```python
from build123d import *

# Parameters (mm, degrees)
CUT_EXTRUDE_1_DEPTH = 2
FILLET_1_R          = 0.2


with BuildPart() as part:
    # 草图1 → 旋转1 (revolve)
    with BuildSketch(Plane.XY):
        Polygon((0, 0), (0, 3.5), (3.5, 3.5), (3.5, 2), (7.5, 2), (7.5, 1.5), (13.5, 1.5), (13.5, 0), align=None)
    revolve(axis=Axis((13.5, 0, 0), (-1, 0, 0)))

    # 草图2 → 切除-拉伸1 (cut)
    with BuildSketch(Plane.ZY):
        Polygon((1.5, 0.866025404), (0, 1.732050808), (-1.5, 0.866025404), (-1.5, -0.866025404), (0, -1.732050808), (1.5, -0.866025404), align=None)
    extrude(amount=-CUT_EXTRUDE_1_DEPTH, mode=Mode.SUBTRACT)

    # 圆角1
    fillet_1_edges = [part.edges().sort_by_distance(p)[0] for p in [
        (3.5, -3.5, 0),
        (0, -3.5, 0),
    ]]
    fillet(fillet_1_edges, radius=FILLET_1_R)


solid = part.part
```
Here's how the part is built. I have some questions about the finished solid (model axes, mm). A direction names the side the tool comes from. Round coordinates to 2 decimals unless told otherwise and drop trailing zeros. Loops run counter-clockwise (first coordinate to the right, second up) from the corner with the lowest first, then second, coordinate; pieces in that order, holes last. Notation, with made-up numbers: (54, 64) -> (75, 64) arc R25 ccw to (75, 103) -> close; hole circle Ø6 at (1.5, 66.25). An arc over 180 degrees is marked (long way). Answer as CSV lines item,"result". Start each with the question number.
1. Imagine slicing it at A-A on x = 1. Write out the boundary of the cut face in (y, z), plus the area to 3 significant figures.
2. I'm going to push flat-ended pins straight in: P1, Ø4, axis at x = 12, y = -1, coming from the +Z side; P2, Ø1, axis at y = 1.5, z = 1.5, coming from the +X side; P3, Ø3, axis at x = 10, y = 1, coming from the -Z side. Where does each tip first touch, or does it pass through?
3. I need wall thicknesses on probe 1 along X at (y, z) = (-0.75, -1.25); probe 2 along X at (y, z) = (0.5, 2.25); probe 3 along Y at (x, z) = (1.25, -1). Which ranges of each line are inside material? Lowest first, please. Write a range as from..to.
4. Imagine slicing it at D-D on x = 5.5. Write out the boundary of the cut face in (y, z).
5. For faces 4 (the face through (10.54, -1.5, -0.07)), 5 (the face through (0.986, 1.305, -0.74)), 6 (the face through (0, 0, -2)), which set-ups out of +Z, -Z, +X, -X, +Y, -Y let a thin tool reach every point of the face, with its end or its side?
6. If we mould it in two halves opening along Z, with no side actions, what happens to faces 1 (the face through (6, 0, 2)), 2 (the face through (2, 0, 0)), 3 (the face through (13.5, 0, 0))? For each: pulls with the +Z half, pulls with the -Z half, needs draft (parallel to the pull), parting line crosses it, or undercut.
7. Imagine slicing it at C-C on x = 10.5. Write out the boundary of the cut face in (y, z).
8. Imagine slicing it at B-B on y = 0. Write out the boundary of the cut face in (x, z).
Solution:
1,outline,"circle Ø7 at (0, 0); hole (-1.73, 0) -> (-0.87, -1.5) -> (0.87, -1.5) -> (1.73, 0) -> (0.87, 1.5) -> (-0.87, 1.5) -> close"
1,area,"30.7 mm²"
2,P1,"z = 1.5"
2,P2,"x = 7.5"
2,P3,"z = -1.5"
3,probe 1,"2..13.5"
3,probe 2,"0..3.5"
3,probe 3,"-3.35..-1.15, 1.15..3.35"
4,outline,"circle Ø4 at (0, 0)"
5,face 4,"+X"
5,face 5,"-X"
5,face 6,"+Z, -Z, -X, +Y, -Y"
6,face 1,"parting line crosses it"
6,face 2,"undercut"
6,face 3,"needs draft"
7,outline,"circle Ø3 at (0, 0)"
8,outline,"(0, -3.3) arc R0.2 ccw to (0.2, -3.5) -> (3.3, -3.5) arc R0.2 ccw to (3.5, -3.3) -> (3.5, -2) -> (7.5, -2) -> (7.5, -1.5) -> (13.5, -1.5) -> (13.5, 1.5) -> (7.5, 1.5) -> (7.5, 2) -> (3.5, 2) -> (3.5, 3.3) arc R0.2 ccw to (3.3, 3.5) -> (0.2, 3.5) arc R0.2 ccw to (0, 3.3) -> (0, 1.5) -> (2, 1.5) -> (2, -1.5) -> (0, -1.5) -> close"
